```python
from build123d import *

# Parameters (mm, degrees)
SALIENTE_EXTRUIR1_DEPTH = 20
CROQUIS2_W              = 12
CROQUIS2_H              = 39
CORTAR_EXTRUIR1_DEPTH   = 39
CORTAR_EXTRUIR2_REACH   = 47
CROQUIS3_R              = 2.75
CORTAR_EXTRUIR3_REACH   = 47
CROQUIS4_R              = 2.75


with BuildPart() as part:
    # Croquis1 → Saliente-Extruir1 (new body)
    with BuildSketch(Plane.XY):
        Polygon((0, 0), (45, 0), (45, 45), (39, 45), (0, 6), align=None)
    extrude(amount=SALIENTE_EXTRUIR1_DEPTH)

    # Croquis2 → Cortar-Extruir1 (cut)
    with BuildSketch(Plane.ZY):
        with Locations((10, 25.5)):
            Rectangle(CROQUIS2_W, CROQUIS2_H)
    extrude(amount=-CORTAR_EXTRUIR1_DEPTH, mode=Mode.SUBTRACT)

    # Croquis3 → Cortar-Extruir2 (cut, up to next)
    with BuildSketch(Plane(origin=(45, 0, 0), x_dir=(0, 0, -1), z_dir=(1, 0, 0)), mode=Mode.PRIVATE) as cortar_extruir2_sk1:
        with Locations((-10, 35)):
            Circle(CROQUIS3_R)
    cortar_extruir2_tool1 = extrude(cortar_extruir2_sk1.sketch, amount=-CORTAR_EXTRUIR2_REACH, mode=Mode.PRIVATE) & part.part
    add(cortar_extruir2_tool1.solids().sort_by_distance((45, 35, 10))[0], mode=Mode.SUBTRACT)
    # Croquis3 → Cortar-Extruir2 (cut, up to next)
    with BuildSketch(Plane(origin=(45, 0, 0), x_dir=(0, 0, -1), z_dir=(1, 0, 0)), mode=Mode.PRIVATE) as cortar_extruir2_sk2:
        with Locations((-10, 19)):
            Circle(CROQUIS3_R)
    cortar_extruir2_tool2 = extrude(cortar_extruir2_sk2.sketch, amount=-CORTAR_EXTRUIR2_REACH, mode=Mode.PRIVATE) & part.part
    add(cortar_extruir2_tool2.solids().sort_by_distance((45, 19, 10))[0], mode=Mode.SUBTRACT)

    # Croquis4 → Cortar-Extruir3 (cut, up to next)
    with BuildSketch(Plane.XZ, mode=Mode.PRIVATE) as cortar_extruir3_sk1:
        with Locations((10, 10)):
            Circle(CROQUIS4_R)
    cortar_extruir3_tool1 = extrude(cortar_extruir3_sk1.sketch, amount=-CORTAR_EXTRUIR3_REACH, mode=Mode.PRIVATE) & part.part
    add(cortar_extruir3_tool1.solids().sort_by_distance((10, 0, 10))[0], mode=Mode.SUBTRACT)
    # Croquis4 → Cortar-Extruir3 (cut, up to next)
    with BuildSketch(Plane.XZ, mode=Mode.PRIVATE) as cortar_extruir3_sk2:
        with Locations((26, 10)):
            Circle(CROQUIS4_R)
    cortar_extruir3_tool2 = extrude(cortar_extruir3_sk2.sketch, amount=-CORTAR_EXTRUIR3_REACH, mode=Mode.PRIVATE) & part.part
    add(cortar_extruir3_tool2.solids().sort_by_distance((26, 0, 10))[0], mode=Mode.SUBTRACT)


solid = part.part
```
The model under review builds one solid part; all positions refer to its coordinate system, in mm. A direction names the side the tool comes from. Round coordinates to 2 decimals unless told otherwise and drop trailing zeros. Write each loop counter-clockwise with the first axis right and the second up, starting at its lowest first coordinate (ties: lowest second). Pieces come first, ordered by that corner, then holes. Notation, with made-up numbers: (12, 15) - (51, 15) arc R11 cw to (51, 31) - close; hole circle Ø5 at (79, 51). An arc over 180 degrees is marked (long way). Use one line per item in the form item = value.
Q1. Consider section B-B (x = 26). State the section outline as (y, z) points, and give its area (3 significant figures).
Answer key:
outline = (0, 0) - (32, 0) - (32, 4) - (6, 4) - (6, 7.25) - (0, 7.25) - close; (0, 12.75) - (6, 12.75) - (6, 16) - (32, 16) - (32, 20) - (0, 20) - close
area = 295 mm2
Q2. Consider section A-A (y = 35). State the section outline as (x, z) points, and give its area (3 significant figures).
Answer key:
outline = (29, 0) - (45, 0) - (45, 7.25) - (39, 7.25) - (39, 4) - (29, 4) - close; (29, 16) - (39, 16) - (39, 12.75) - (45, 12.75) - (45, 20) - (29, 20) - close
area = 167 mm2
Q3. Draft analysis for pull direction X (two halves, no side actions). For faces 1 (the flat face through (39, 26, 10)), 2 (the flat face through (27, 18, 20)), 3 (the cylindrical face through (11.48, 2.96, 12.32)), state which applies: +X half, -X half, draft (parallel to the pull), parting line (faces both ways), or undercut.
Answer key:
face_1 = -X half
face_2 = draft
face_3 = undercut
Q4. Consider section D-D (x = 37.5). State the section outline as (y, z) points, and give its area (3 significant figures).
Answer key:
outline = (0, 0) - (43.5, 0) - (43.5, 4) - (6, 4) - (6, 16) - (43.5, 16) - (43.5, 20) - (0, 20) - close
area = 420 mm2
Q5. Insertion check: pin 1 Ø3.5 at (x, z) = (12, 7) entering from +Y; pin 2 Ø3.5 at (y, z) = (21, 10) entering from -X; pin 3 Ø12 at (x, z) = (18.5, 11.5) entering from +Y. Each pin has a flat end and moves straight along its axis. Give the tip position at first contact, or say it passes through.
Answer key:
pin_1 = 6
pin_2 = 39
pin_3 = 28.47
Q6. For line 1 (Y direction, x = 41.85, z = 10); line 2 (Z direction, x = 31.5, y = 22); line 3 (X direction, y = 5, z = 10.75), list the stretches that pass through material, from the lowest coordinate up. Write a range as [from, to].
Answer key:
line_1 = [0, 16.25], [21.75, 32.25], [37.75, 45]
line_2 = [0, 4], [16, 20]
line_3 = [0, 7.35], [12.65, 23.35], [28.65, 45]
Q7. Tool access review of faces 4 (the cylindrical face through (42.042, 21.727, 10.358)), 5 (the flat face through (19, 6, 10)): name each direction out of +Z, -Z, +X, -X, +Y, -Y from which nothing blocks a thin tool from reaching the whole face with its end or side.
Answer key:
face_4 = +X, -X
face_5 = -X, +Y
Q8. Consider section C-C (z = 10). State the section outline as (x, y) points.
Answer key:
outline = (0, 0) - (7.25, 0) - (7.25, 6) - (0, 6) - close; (12.75, 0) - (23.25, 0) - (23.25, 6) - (12.75, 6) - close; (28.75, 0) - (45, 0) - (45, 16.25) - (39, 16.25) - (39, 6) - (28.75, 6) - close; (39, 21.75) - (45, 21.75) - (45, 32.25) - (39, 32.25) - close; (39, 37.75) - (45, 37.75) - (45, 45) - (39, 45) - close
